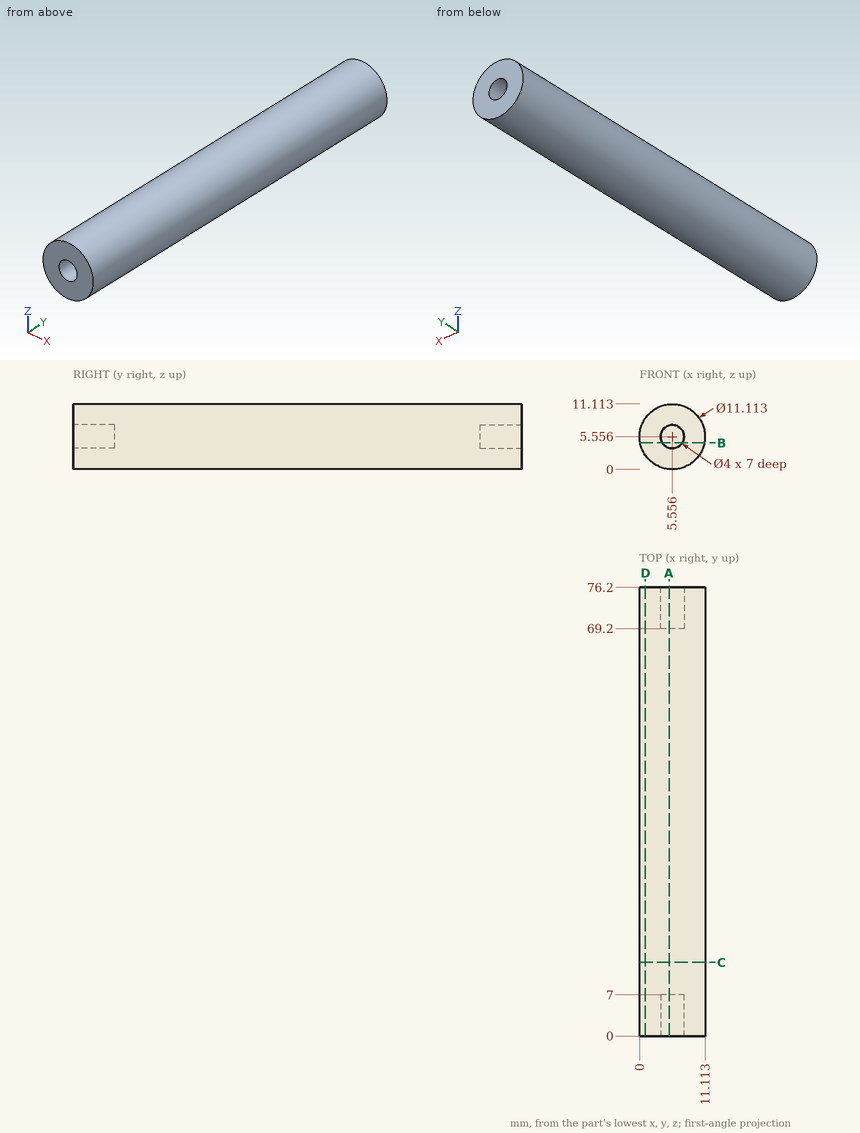
Answer from the drawing. Dimensions are ordinates in mm from the lowest x, y and z of the part. Give positions to 0.01 mm unless a question says otherwise; leave off trailing zeros. Write each loop counter-clockwise with the first axis right and the second up, starting at its lowest first coordinate (ties: lowest second). Pieces come first, ordered by that corner, then holes. Notation, with made-up numbers: (28, -0.5) -> (43, -0.5) arc R23 cw to (43, 37.5) -> close; hole circle Ø5 at (29.25, -20). An arc over 180 degrees is marked (long way). One line per question, with ' | ' between items. Start each with the question number.
1. Section C-C (y = 12.5) is taken. Determine the outline of the cut face in (x, z), plus the area to 3 significant figures.
2. Section B-B (z = 4.5) is taken. Determine the outline of the cut face in (x, y) (1 decimal).
3. Section A-A (x = 5) is taken. Determine the outline of the cut face in (y, z) (1 decimal).
4. Given pin 1 Ø2 at (x, z) = (6, 5.5) entering from +Y; pin 2 Ø1 at (y, z) = (58.5, 8) entering from +X, each flat-ended and moving along its own axis, determine where each tip first touches the part or whether it passes through.
5. Section D-D (x = 1) is taken. Determine the outline of the cut face in (y, z), plus the area to 3 significant figures.
6. Find the intervals of material crossed by probe 1 along Y at (x, z) = (5.5, 5.25); probe 2 along Z at (x, y) = (5.25, 22) (1 decimal); probe 3 along Z at (x, y) = (4, 17), in increasing order.
Response values:
1) outline: circle Ø11.11 at (5.56, 5.56) | area: 97.0 mm2
2) outline: (0.1, 0) -> (3.9, 0) -> (3.9, 7) -> (7.3, 7) -> (7.3, 0) -> (11, 0) -> (11, 76.2) -> (7.3, 76.2) -> (7.3, 69.2) -> (3.9, 69.2) -> (3.9, 76.2) -> (0.1, 76.2) -> close
3) outline: (0, 0) -> (76.2, 0) -> (76.2, 3.6) -> (69.2, 3.6) -> (69.2, 7.5) -> (76.2, 7.5) -> (76.2, 11.1) -> (0, 11.1) -> (0, 7.5) -> (7, 7.5) -> (7, 3.6) -> (0, 3.6) -> close
4) pin 1: y = 69.2 | pin 2: x = 10.76
5) outline: (0, 2.38) -> (76.2, 2.38) -> (76.2, 8.74) -> (0, 8.74) -> close | area: 485 mm2
6) probe 1: 7 to 69.2 | probe 2: 0 to 11.1 | probe 3: 0.22 to 10.89
